Can you work these out from the model? Positions are in its coordinate system, mm. A direction names the side the tool comes from. Round coordinates to 2 decimals unless told otherwise and drop trailing zeros. Loops run counter-clockwise (first coordinate to the right, second up) from the corner with the lowest first, then second, coordinate; pieces in that order, holes last.
from build123d import *

# Parameters (mm, degrees)
SKETCH1_R           = 75
BOSS_EXTRUDE1_DEPTH = 3.175
SKETCH2_W           = 54.82616321
SKETCH2_H           = 7.62
CUT_EXTRUDE1_DEPTH  = 3.175
SKETCH4_R           = 1.5875
CUT_EXTRUDE2_DEPTH  = 3.175
SKETCH5_W           = 6.096
SKETCH5_H           = 3.175
CUT_EXTRUDE3_DEPTH  = 3.175
SKETCH6_R           = 1.016
CUT_EXTRUDE4_DEPTH  = 3.175


with BuildPart() as part:
    # Sketch1 → Boss-Extrude1 (new body)
    with BuildSketch(Plane(origin=(0, 0, 0), x_dir=(1, 0, 0), z_dir=(0, 1, 0))):
        Circle(SKETCH1_R)
    extrude(amount=BOSS_EXTRUDE1_DEPTH)

    # Sketch2 → Cut-Extrude1 (cut)
    with BuildSketch(Plane(origin=(0, 3.175, 0), x_dir=(1, 0, 0), z_dir=(0, 1, 0))):
        with Locations((0, 59.129220339)):
            Rectangle(SKETCH2_W, SKETCH2_H)
        with Locations((0, -59.129220339)):
            Rectangle(SKETCH2_W, SKETCH2_H)
    extrude(amount=-CUT_EXTRUDE1_DEPTH, mode=Mode.SUBTRACT)

    # Sketch4 → Cut-Extrude2 (cut)
    with BuildSketch(Plane(origin=(0, 3.175, 0), x_dir=(1, 0, 0), z_dir=(0, 1, 0))):
        with Locations((-52.180304588, 44.729838125)):
            Circle(SKETCH4_R)
        with Locations((-19.05, 44.729838125)):
            Circle(SKETCH4_R)
        with Locations((-60.791780161, 34.29)):
            Circle(SKETCH4_R)
        with Locations((-17.611780161, 34.29)):
            Circle(SKETCH4_R)
        with Locations((-60.791780161, -34.29)):
            Circle(SKETCH4_R)
        with Locations((-52.180304588, -44.729838125)):
            Circle(SKETCH4_R)
        with Locations((-17.611780161, -34.29)):
            Circle(SKETCH4_R)
        with Locations((-19.05, -44.729838125)):
            Circle(SKETCH4_R)
        with Locations((17.611780161, -34.29)):
            Circle(SKETCH4_R)
        with Locations((19.05, -44.729838125)):
            Circle(SKETCH4_R)
        with Locations((52.180304588, -44.729838125)):
            Circle(SKETCH4_R)
        with Locations((60.791780161, -34.29)):
            Circle(SKETCH4_R)
        with Locations((60.791780161, 34.29)):
            Circle(SKETCH4_R)
        with Locations((52.180304588, 44.729838125)):
            Circle(SKETCH4_R)
        with Locations((19.05, 44.729838125)):
            Circle(SKETCH4_R)
        with Locations((17.611780161, 34.29)):
            Circle(SKETCH4_R)
        with Locations((0, 11.494220339)):
            Circle(SKETCH4_R)
        with Locations((0, -11.494220339)):
            Circle(SKETCH4_R)
    extrude(amount=-CUT_EXTRUDE2_DEPTH, mode=Mode.SUBTRACT)

    # Sketch5 → Cut-Extrude3 (cut)
    with BuildSketch(Plane(origin=(0, 3.175, 0), x_dir=(1, 0, 0), z_dir=(0, 1, 0))):
        with Locations((64.732085553, 22.86)):
            Rectangle(SKETCH5_W, SKETCH5_H)
        with Locations((64.732085553, -22.86)):
            Rectangle(SKETCH5_W, SKETCH5_H)
        with Locations((-64.732085553, -22.86)):
            Rectangle(SKETCH5_W, SKETCH5_H)
        with Locations((-64.732085553, 22.86)):
            Rectangle(SKETCH5_W, SKETCH5_H)
        Polygon((39.817492218, 59.646380223), (42.418494964, 57.825553566), (38.922507782, 52.831628294), (36.321505036, 54.652454951), align=None)
        Polygon((38.922507782, -52.831628294), (42.418494964, -57.825553566), (39.817492218, -59.646380223), (36.321505036, -54.652454951), align=None)
        Polygon((-38.922507782, -52.831628294), (-36.321505036, -54.652454951), (-39.817492218, -59.646380223), (-42.418494964, -57.825553566), align=None)
        Polygon((-39.817492218, 59.646380223), (-36.321505036, 54.652454951), (-38.922507782, 52.831628294), (-42.418494964, 57.825553566), align=None)
    extrude(amount=-CUT_EXTRUDE3_DEPTH, mode=Mode.SUBTRACT)

    # Sketch6 → Cut-Extrude4 (cut)
    with BuildSketch(Plane(origin=(0, 3.175, 0), x_dir=(1, 0, 0), z_dir=(0, 1, 0))):
        with Locations((50.8, 6.731)):
            Circle(SKETCH6_R)
        with Locations((50.8, -6.731)):
            Circle(SKETCH6_R)
    cut_extrude4 = extrude(amount=-CUT_EXTRUDE4_DEPTH, mode=Mode.SUBTRACT)

    # Mirror1: Cut-Extrude4 across plane
    add(cut_extrude4.mirror(Plane(origin=(0, 0, 0), x_dir=(0, 0, 1), z_dir=(1, 0, 0))), mode=Mode.SUBTRACT)


solid = part.part
(1) If I drill on line 1 (Z direction, x = 0, y = 1.15); line 2 (X direction, y = 1.15, z = -34.5); line 3 (X direction, y = 1.8, z = -45.5), over which ranges is the centre line in solid material (lowest first)?
Worked answers:
line 1: z = -75 to -62.94, -55.32 to -13.08, -9.91 to 9.91, 13.08 to 55.32, 62.94 to 75
line 2: x = -66.59 to -62.37, -59.22 to -19.19, -16.04 to 16.04, 19.19 to 59.22, 62.37 to 66.59
line 3: x = -59.62 to -53.57, -50.79 to -20.44, -17.66 to 17.66, 20.44 to 50.79, 53.57 to 59.62
(2) If we section it at C-C, the plane z = -50.5: List the corners of the cut face in (x, y) for me (3 decimals), then the cut area to 3 significant figures.
Worked answers:
outline: (-55.45, 0) - (55.45, 0) - (55.45, 3.175) - (-55.45, 3.175) - close
area: 352 mm2
(3) If we mould it in two halves opening along Z, with no side actions, what happens to faces 3 (the cylindrical face through (-9.764, 1.565, -74.362)), 4 (the flat face through (38.045, 1.61, -57.114)), 5 (the flat face through (-1, 3.175, -1))? For each: released by +Z, released by -Z, zero draft, split by the parting line, or undercut.
Worked answers:
face 3: split by the parting line
face 4: undercut
face 5: zero draft
(4) For faces 1 (the flat face through (-1, 0, -1)), 2 (the flat face through (38.09, 1.61, 57.18)), which set-ups out of +Z, -Z, +X, -X, +Y, -Y let a thin tool reach every point of the face, with its end or its side?
Worked answers:
face 1: +Z, -Z, +X, -X, -Y
face 2: +Y, -Y
(5) If we section it at A-A, the plane y = 1.75: State how many separate pieces and enclosed holes the cut face has, then the cut area to 3 significant figures.
Worked answers:
separate pieces: 1
enclosed holes: 32
area: 16,500 mm2
(6) Will these pins go through, and if not, where does the flat tip stop? P1, Ø1.5, axis at y = 2, z = -48, coming from the -X side; P2, Ø1, axis at y = 1, z = 59, coming from the +X side; P3, Ø1, axis at y = 2.5, z = -31.5, coming from the -X side.
Worked answers:
P1: stops at x = -58.24
P2: stops at x = 46.93
P3: stops at x = -68.29
(7) If we section it at B-B, the plane x = 46: List the corners of the cut face in (y, z) for me (3 decimals), then the cut area to 3 significant figures.
Worked answers:
outline: (0, -59.237) - (3.175, -59.237) - (3.175, 59.237) - (0, 59.237) - close
area: 376 mm2
